Autodesk Fusion 360 part; units mm, degrees
sketch "Sketch1" plane through (0, 0, 0) normal (1, 0, 0) x (0, 1, 0)
  line L0 (0, 80) -> (0, -40) construction
  line L1 (0, 0) -> (45, 0)
  line L2 (45, 0) -> (45, 1)
  line L3 (0, 0) -> (0, 20) construction
  line L4 (0, 20) -> (1.5, 20)
  line L5 (44, 2) -> (15, 2)
  spline S0 degree 2 poles (1.5, 20) (4.0396, 7.8722) (15, 2) knots 0 0 0 2.340033 2.340033 2.340033 weights 1 1.582771 1
  arc A0 (45, 1) -> (44, 2) centre (44, 1) ccw
  line L6 (0, 20) -> (0, 0) construction
  line L7 (0, 20) -> (0, 0)
  point P0 (45, 2)
  dimension "d1" = 120
  dimension "d2" = 45
  dimension "d3" = 2
  dimension "d4" = 20
  dimension "d5" = 1.5
  dimension "d6" = 30
  dimension "d7" = 1
revolve "Revolve1" add sketch "Sketch1" angle 360 about axis through (0, 0, 20) along (0, 0, -1)
fillet "Fillet1" radius 0.5 1 edges at (-1.3985, 0.5424, 20)
sketch "Sketch2" plane through (0, 0, 2) normal (0, 0, 1) x (-1, 0, 0)
  circle A0 centre (0, 0) radius 15
  circle A1 centre (0, 0) radius 44
  circle A2 centre (0, 0) radius 30 construction
  line L0 (0, 0) -> (25, 25) construction
  line L1 (0, 0) -> (-21.2132, -21.2132) construction
  line L2 (0, 0) -> (-22.657, 22.657) construction
  line L3 (0, 0) -> (23.9132, -23.9132) construction
  circle A3 centre (21.2132, -21.2132) radius 4
  circle A4 centre (-21.2132, -21.2132) radius 4
  circle A5 centre (21.2132, 21.2132) radius 4
  circle A6 centre (-21.2132, 21.2132) radius 4
  circle A7 centre (21.2132, -21.2132) radius 2.6
  circle A8 centre (-21.2132, -21.2132) radius 2.6
  circle A9 centre (-21.2132, 21.2132) radius 2.6
  circle A10 centre (21.2132, 21.2132) radius 2.6
  circle A11 centre (10.6066, -10.6066) radius 5
  dimension "d11" = 60
  dimension "d12" = 35.3553
  dimension "d13" = 30
  dimension "d14" = 32.0419
  dimension "d15" = 33.8184
  dimension "d16" = 8
  dimension "d17" = 8
  dimension "d18" = 8
  dimension "d19" = 8
  dimension "d20" = 5.2
  dimension "d21" = 5.2
  dimension "d22" = 5.2
  dimension "d23" = 5.2
  dimension "d31" = 10
  dimension "d34" = 15
extrude "Extrude3" add sketch "Sketch2" along normal blind 8 contours A3 | A4 | A5 | A6
extrude "Extrude2" cut sketch "Sketch2" against normal blind 5 contours A7 | A8 | A9 | A10
extrude "Extrude4" cut sketch "Sketch2" along normal mid plane 18 contours A0 A11 | A0 A11 picked at (9.3285, -9.5024) picked at (11.819, -11.7173)
Input: part model. Units: mm. Frame: model coordinates. A direction names the side the tool comes from. Coordinates: 2 decimals unless noted, no trailing zeros. Put each result on its own line as item: value.
1. Cut plane A-A on z = 7.5. State how many separate pieces and enclosed holes the cut face has, then the cut area to 3 significant figures.
Report:
separate pieces: 5
enclosed holes: 4
area: 272 mm2
2. Reachability of faces 4 (the face through (-24, -21, 10)), 5 (the face through (-23.059, 17.665, 5.944)) from +Z, -Z, +X, -X, +Y, -Y: full face, straight path, thin tool, end or side. Return the list, or none.
Report:
face 4: +Z, +X, -X, +Y, -Y
face 5: +Z
3. Contact query for flat-ended pins moving along their axis: pin 1 Ø12 at (x, y) = (-19.5, -18) entering from -Z; pin 2 Ø4 at (x, z) = (23.5, 10) entering from +Y; pin 3 Ø4 at (x, y) = (-21.21, 21.21) entering from -Z; pin 4 Ø4 at (x, y) = (-22.5, -22) entering from +Z. Output: stop coordinate, or through.
Report:
pin 1: stops at z = 0
pin 2: stops at y = 25.2
pin 3: passes through
pin 4: stops at z = 10
4. Line query: line 1 along X through (y, z) = (19.5, 9); line 2 along Y through (x, z) = (-1, 18.25); line 3 along Z through (x, y) = (-41, -11.5). Output: solid intervals per line, ascending.
Report:
line 1: x = -24.83 to -23.17, -19.26 to -17.6, 17.6 to 19.26, 23.17 to 24.83
line 2: y = -1.6 to 1.6
line 3: z = 0 to 2
5. Draft query along Y for faces 1 (the face through (22.08, 17.31, 5.94)), 2 (the face through (-21, 24, 10)), 3 (the face through (39.923, 20.765, 0.507)). Return one class per face: pulls with the +Y half, pulls with the -Y half, needs draft (parallel to the pull), parting line crosses it, or undercut.
Report:
face 1: undercut
face 2: needs draft
face 3: parting line crosses it
